from build123d import *

# Parameters (mm, degrees)
BOSS_EXTRUDE1_START = 9
SKETCH3_R           = 4.25
BOSS_EXTRUDE1_DEPTH = 9
CIRPATTERN1_COUNT   = 3
SKETCH4_R           = 5
BOSS_EXTRUDE2_DEPTH = 12.7


with BuildPart() as part:
    # Sketch1 → Revolve1 (revolve)
    with BuildSketch(Plane.XY, mode=Mode.PRIVATE) as revolve1_sk:
        Polygon((0, 78.640438678), (0, -19.887292524), (16, -19.887292524), (16, -11.949792524), (30.1625, -11.949792524), (39.6875, -2.424792524), (39.6875, 6.694938678), (50.5, 6.694938678), (50.5, 16.219938678), (50.246, 16.219938678), (50.246, 16.473938678), (50.5, 16.473938678), (50.5, 78.386438678), (50.246, 78.386438678), (50.246, 78.640438678), align=None)
    revolve(revolve1_sk.sketch.rotate(Axis((0, -28.529868613, 0), (0, 1, 0)), 90), axis=Axis((0, -28.529868613, 0), (0, 1, 0)))

    # Sketch3 → Boss-Extrude1 (add)
    with BuildSketch(Plane(origin=(0, 78.640438678, 0), x_dir=(1, 0, 0), z_dir=(0, 1, 0)).offset(BOSS_EXTRUDE1_START)):
        with BuildLine():
            Line((-8.246317561, 56.400339065), (-8.527789484, 54.9019935))
            ThreePointArc((-8.527789484, 54.9019935), (-10.543132136, 50.831813425), (-14.384179724, 48.408112685))
            ThreePointArc((-14.384179724, 48.408112685), (0, -50.5), (14.384179724, 48.408112685))
            ThreePointArc((14.384179724, 48.408112685), (10.543132136, 50.831813425), (8.527789484, 54.9019935))
            Line((8.527789484, 54.9019935), (8.246317561, 56.400339065))
            ThreePointArc((8.246317561, 56.400339065), (0, 63.241786356), (-8.246317561, 56.400339065))
        make_face()
        with Locations(Location((0, 57, 0), (0, 0, 270))):
            Circle(SKETCH3_R, mode=Mode.SUBTRACT)
    boss_extrude1 = extrude(amount=-BOSS_EXTRUDE1_DEPTH)

    # CirPattern1: Boss-Extrude1 ×3 about axis
    cirpattern1_axis = Axis((0, 0, 0), (0, 1, 0))
    for i in range(1, CIRPATTERN1_COUNT):
        add(boss_extrude1.rotate(cirpattern1_axis, i * 360 / CIRPATTERN1_COUNT))

    # Sketch4 → Boss-Extrude2 (add)
    with BuildSketch(Plane(origin=(0, 87.640438678, 0), x_dir=(1, 0, 0), z_dir=(0, 1, 0))):
        with Locations(Location((0, 0, 0), (0, 0, 90))):
            Circle(SKETCH4_R)
    extrude(amount=BOSS_EXTRUDE2_DEPTH)


solid = part.part
Can you work these out from the model? Positions are in its coordinate system, mm. A direction names the side the tool comes from. Coordinates: 2 decimals unless noted, no trailing zeros. Order: outer loops, then holes, each group sorted by start corner. A loop starts at its lowest first (then second) coordinate and runs counter-clockwise, first axis right, second up. Notation, with made-up numbers: M 73.25,-8 L 103.25,-8 A19 ccw 103.25,23 Z; hole C -28.5,89 d2. An arc over 180 degrees is marked long. Answer as CSV lines item,"result".
(1) I'm going to push flat-ended pins straight in: pin 1 (5 mm diameter, centred on x = -30, y = 69.5, fed in from +Z); pin 2 (10 mm diameter, centred on y = 63, z = -20.5, fed in from -X); pin 3 (7 mm diameter, centred on x = -49.36, z = 28.5, fed in from -Y); pin 4 (12 mm diameter, centred on x = 36, y = -2, fed in from +Z). Where does each tip first touch, or does it pass through?
Geometry check:
pin 1,"z = 42.36"
pin 2,"x = -48.06"
pin 3,"through"
pin 4,"z = 25.98"
(2) Please list where these lines run through material, in increasing order: L1, parallel to X at y = 82, z = 28; L2, parallel to X at y = 84.5, z = 28.5; L3, parallel to Y at x = 40.5, z = 15.
Geometry check:
L1,"-55.87 to -53.58, -45.14 to 45.14, 53.58 to 55.87"
L2,"-55.82 to -53.61, -45.11 to 45.11, 53.61 to 55.82"
L3,"6.69 to 87.64"
(3) Suppose I cut it at C-C on z = 28.5. Count the separate pieces of the cut face and the enclosed holes in it, plus the area to 3 significant figures.
Geometry check:
separate pieces,"3"
enclosed holes,"0"
area,"7,730 mm^2"
(4) On a 3-axis mill with a long thin cutter (end or side, diameter ignored), from which of +Z, -Z, +X, -X, +Y, -Y can I reach the whole of each face in a straight line? I mean faces 1 (the cylindrical face through (45.593, 83.203, 30.461)), 2 (the cylindrical face through (-0.536, 83.203, 50.497)), 3 (the flat face through (-42, 78.64, 28)), 4 (the cylindrical face through (-11.921, 2.199, -37.855)), 5 (the cylindrical face through (4.88, 93.9, 1.08)). Say none if no direction works.
Geometry check:
face 1,"+Y, -Y"
face 2,"+Z, +Y, -Y"
face 3,"none"
face 4,"-Y"
face 5,"+Y"
(5) Suppose I cut it at B-B on y = 59. Please give me the cut outline in (x, z).
Geometry check:
outline,"C 0,0 d101"
(6) If we mould it in two halves opening along Y, with no side actions, what happens to faces 6 (the cylindrical face through (-54.85, 83.2, 31.48)), 7 (the flat face through (-4.3, 87.64, -3.4)), 8 (the flat face through (13, -11.95, 13))? For each: released by +Y, released by -Y, zero draft, split by the parting line, or undercut.
Geometry check:
face 6,"zero draft"
face 7,"released by +Y"
face 8,"released by -Y"
